Part print with two shaded views. Sizes in mm from the minimum x, y, z corner. A direction names the side the tool comes from. Round coordinates to 2 decimals unless told otherwise and drop trailing zeros. Order: outer loops, then holes, each group sorted by start corner. A loop starts at its lowest first (then second) coordinate and runs counter-clockwise, first axis right, second up. Notation, with made-up numbers: M 28,-18 L 86,-18 A19 cw 86,5 Z; hole C 18,-17 d8. An arc over 180 degrees is marked long. Put each result on its own line as item: value.
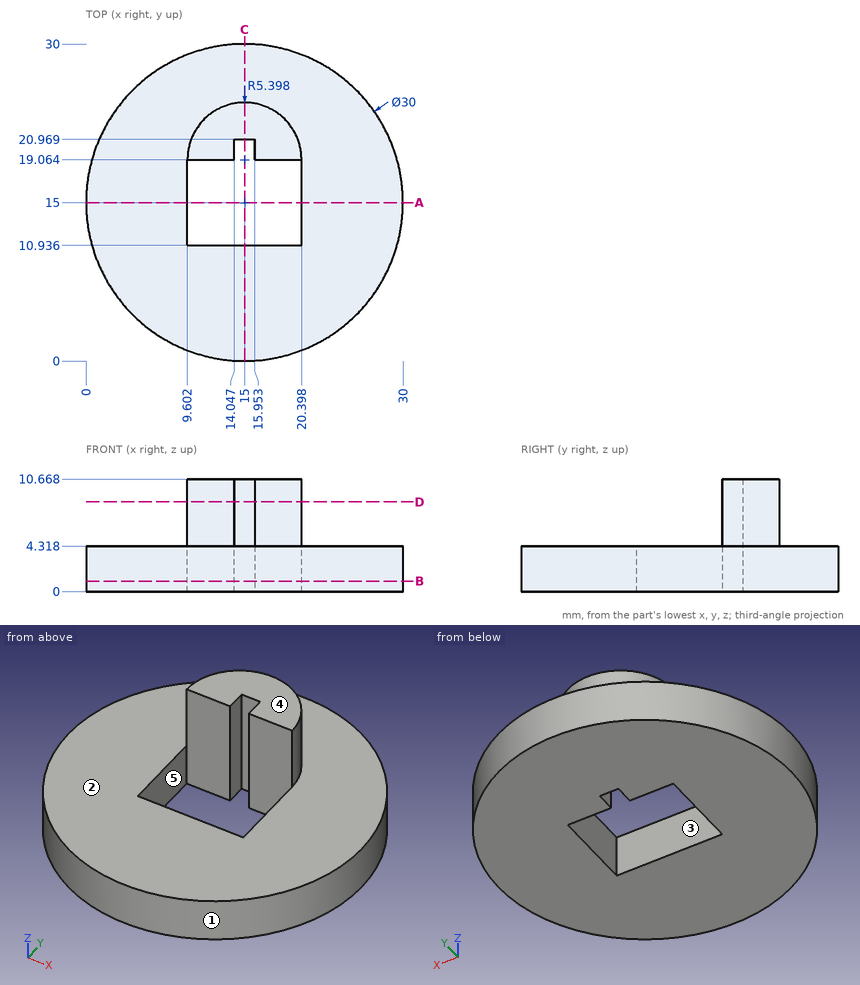
Item 1: Mould opens along X. For the marked faces 1, 2 and 3 say: pulls with the +X half, pulls with the -X half, needs draft (parallel to the pull), parting line crosses it, or undercut.
Answers below:
face 1: parting line crosses it
face 2: needs draft
face 3: undercut
Item 2: Band-saw the part on D-D on z = 8.5. Give the cut face in (x, y) (1 decimal).
Answers below:
outline: M 9.6,19.1 L 14,19.1 L 14,21 L 16,21 L 16,19.1 L 20.4,19.1 A5.4 ccw Z
Item 3: Band-saw the part on A-A on y = 15. Give the cut face in (x, z).
Answers below:
outline: M 0,0 L 9.6,0 L 9.6,4.32 L 0,4.32 Z; M 20.4,0 L 30,0 L 30,4.32 L 20.4,4.32 Z
Item 4: Band-saw the part on C-C on x = 15. Give the cut face in (y, z) (1 decimal), and give its area (3 significant figures).
Answers below:
outline: M 0,0 L 10.9,0 L 10.9,4.3 L 0,4.3 Z; M 21,0 L 30,0 L 30,4.3 L 24.5,4.3 L 24.5,10.7 L 21,10.7 Z
area: 108 mm²
Item 5: Probe line 1 along Z through (x, y) = (21.75, 4.5); line 2 along X through (y, z) = (17, 3) (1 decimal); line 3 along X through (y, z) = (11.25, 0.75) (1 decimal). List the from-to ranges inside material, lowest first. Write a range as [from, to].
Answers below:
line 1: [0, 4.32]
line 2: [0.1, 9.6], [20.4, 29.9]
line 3: [0.5, 9.6], [20.4, 29.5]
Item 6: Tool access for the marked faces 4 and 5: list every direction of +Z, -Z, +X, -X, +Y, -Y with a clear straight run to the whole face (end or side of a thin tool).
Answers below:
face 4: +Z, +X, -X, +Y, -Y
face 5: +Z, -Z
Item 7: Pin check, flat tips, straight feed: P1, Ø3.5, axis at x = 11, z = 7.5, coming from the -Y side; P2, Ø1.5, axis at x = 11, z = 2, coming from the -Y side; P3, Ø6, axis at x = 8, y = 27, coming from the -Z side; P4, Ø2, axis at y = 20, z = 7, coming from the +X side. Stop position of each tip, or through.
Answers below:
P1: y = 19.06
P2: y = 0.36
P3: z = 0
P4: x = 20.4
Item 8: Band-saw the part on B-B on z = 1. Give the cut face in (x, y) (1 decimal).
Answers below:
outline: C 15,15 d30; hole M 9.6,10.9 L 20.4,10.9 L 20.4,19.1 L 16,19.1 L 16,21 L 14,21 L 14,19.1 L 9.6,19.1 Z
